Could you check a few things on this drawing? It's one solid part, dimensions in mm from its lowest x, y, z. A direction names the side the tool comes from. Give positions to 0.01 mm unless a question says otherwise; leave off trailing zeros. Loops run counter-clockwise (first coordinate to the right, second up) from the corner with the lowest first, then second, coordinate; pieces in that order, holes last. Notation, with made-up numbers: (-24.5, -6) - (28.5, -6) arc R21 cw to (28.5, 0) - close; hole circle Ø2 at (-23, 89.5). An arc over 180 degrees is marked (long way). Answer as a JSON object with one key per item and string values.
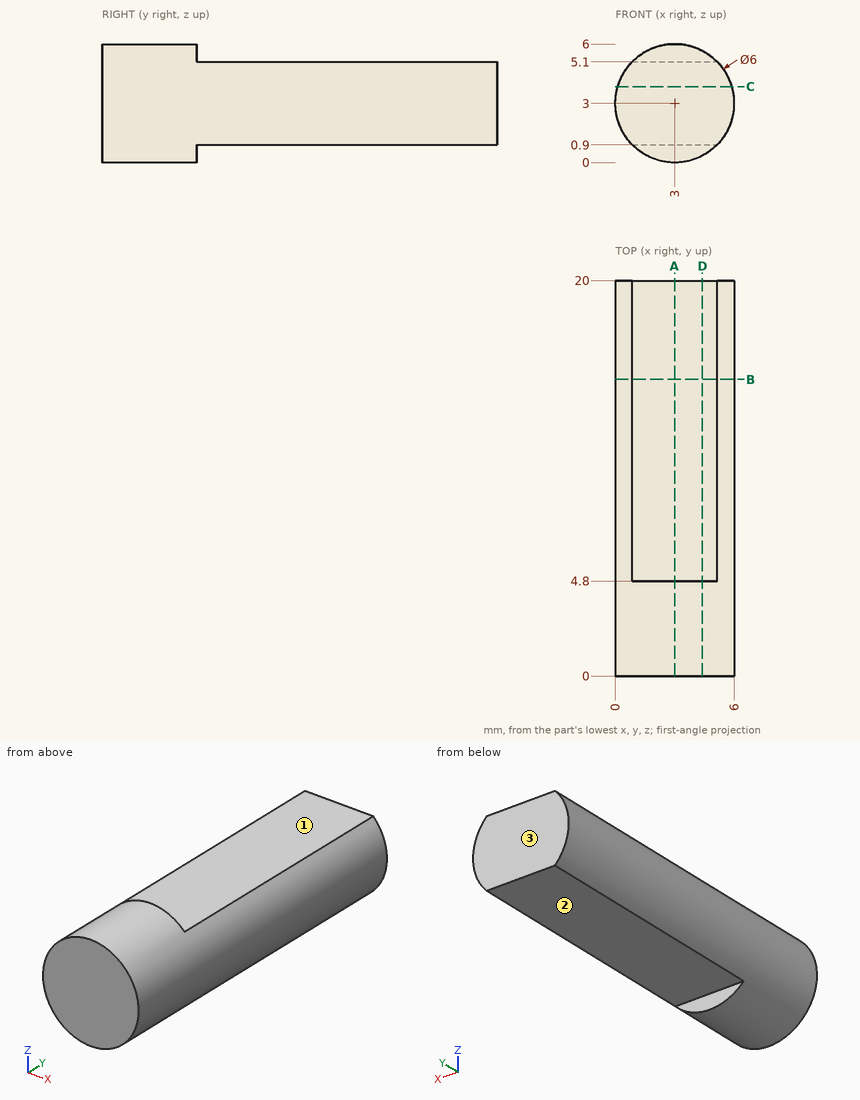
1) Imagine slicing it at B-B on y = 15. Write out the boundary of the cut face in (x, z), and give its area (3 significant figures).
Check sheet entries:
{"outline": "(0.86, 0.9) - (5.14, 0.9) arc R3 ccw to (5.14, 5.1) - (0.86, 5.1) arc R3 ccw to start", "area": "23.0 mm2"}
2) Imagine slicing it at A-A on x = 3. Write out the boundary of the cut face in (y, z), and give its area (3 significant figures).
Check sheet entries:
{"outline": "(0, 0) - (4.8, 0) - (4.8, 0.9) - (20, 0.9) - (20, 5.1) - (4.8, 5.1) - (4.8, 6) - (0, 6) - close", "area": "92.6 mm2"}
3) I need wall thicknesses on L1, parallel to Z at x = 2.1, y = 15.5; L2, parallel to X at y = 6.5, z = 4.6; L3, parallel to X at y = 7.25, z = 4.3. Which ranges of each line are inside material? Lowest first, please.
Check sheet entries:
{"L1": "0.9 to 5.1", "L2": "0.46 to 5.54", "L3": "0.3 to 5.7"}
4) Which directions (+Z, -Z, +X, -X, +Y, -Y) give clear straight access to the entire face, cutting with the end or side of a thin tool? Please do the marked faces 1, 2 and 3.
Check sheet entries:
{"face 1": "+Z, +X, -X, +Y", "face 2": "-Z, +X, -X, +Y", "face 3": "+Z, -Z, +X, -X, +Y"}
5) I'm going to push flat-ended pins straight in: P1, Ø2, axis at x = 3, y = 15, coming from the -Z side; P2, Ø2, axis at x = 1, y = 2, coming from the +Z side; P3, Ø0.7, axis at x = 3.5, z = 5.5, coming from the +Y side; P4, Ø1, axis at x = 3, z = 0.5, coming from the +Y side. Where does each tip first touch, or does it pass through?
Check sheet entries:
{"P1": "z = 0.9", "P2": "z = 5.83", "P3": "y = 4.8", "P4": "y = 20"}
6) Imagine slicing it at C-C on z = 3.85. Write out the boundary of the cut face in (x, y), and give its area (3 significant figures).
Check sheet entries:
{"outline": "(0.12, 0) - (5.88, 0) - (5.88, 20) - (0.12, 20) - close", "area": "115 mm2"}
7) Imagine slicing it at D-D on x = 4.4. Write out the boundary of the cut face in (y, z).
Check sheet entries:
{"outline": "(0, 0.35) - (4.8, 0.35) - (4.8, 0.9) - (20, 0.9) - (20, 5.1) - (4.8, 5.1) - (4.8, 5.65) - (0, 5.65) - close"}
